```python
from build123d import *

# Parameters (mm, degrees)
F1_DEPTH  = 7.89
F3_DEPTH  = 9
F4_R      = 1.55
F5_DEPTH  = 25
F6_DEPTH  = 33
F7_R      = 2.53
F7_R_2    = 1.55
F8_DEPTH  = 1.12
F10_DEPTH = 1.98
F11_W     = 5.31
F11_H     = 0.8
F12_DEPTH = 1
F13_W     = 4.8969178084
F13_H     = 5.51
F14_DEPTH = 5.97
F15_R     = 2.46
F16_DEPTH = 2.5


with BuildPart() as f1:
    # F0 (on Front) → F1 (new body)
    with BuildSketch(Plane.XZ):
        Polygon((0, 10.28), (0, 1.53), (1.3, 1.53), (1.3, 2.33), (6.61, 2.33), (6.61, 1.53), (7.91, 1.53), (7.91, 10.28), align=None)
    extrude(amount=F1_DEPTH)

    # F2 (on face) → F3 (join)
    with BuildSketch(Plane.XZ.offset(7.89)):
        Polygon((1.3, 1.53), (0, 1.53), (0, 0), (7.91, 0), (7.91, 1.53), (6.61, 1.53), align=None)
    extrude(amount=-F3_DEPTH)

    # F4 (on face) → F5 (join)
    with BuildSketch(Plane(origin=(0, 0, 0), x_dir=(-1, 0, 0), z_dir=(0, 1, 0))):
        with Locations((-3.955, 6.065)):
            Circle(F4_R)
    extrude(amount=F5_DEPTH)

    # F6 (cut): a face of the model
    f6_faces = [f1.faces().sort_by_distance(p)[0] for p in [
        (3.955, 25, 6.065),
    ]]
    extrude(f6_faces, amount=-F6_DEPTH, mode=Mode.SUBTRACT)

    # F7 (on face) → F8 (join)
    with BuildSketch(Plane(origin=(0, 0, 0), x_dir=(-1, 0, 0), z_dir=(0, 1, 0))):
        with Locations((-3.955, 6.065)):
            Circle(F7_R)
        with Locations((-3.955, 6.065)):
            Circle(F7_R_2, mode=Mode.SUBTRACT)
    extrude(amount=F8_DEPTH)

    # F9 (on face) → F10 (join)
    with BuildSketch(Plane.XY.offset(10.28)):
        with BuildLine():
            ThreePointArc((3.955, 0), (2.487753429, -3.542246571), (6.03, -2.075))
            ThreePointArc((6.03, -2.075), (5.422246571, -0.607753429), (3.955, 0))
        make_face()
    extrude(amount=F10_DEPTH)

    # F11 (on face) → F12 (join)
    with BuildSketch(Plane.XZ.offset(7.89)):
        with Locations((3.955, 1.93)):
            Rectangle(F11_W, F11_H)
    extrude(amount=-F12_DEPTH)

    # F13 (on face) → F14 (cut)
    with BuildSketch(Plane.XZ.offset(7.89)):
        with Locations((3.955, 5.935)):
            Rectangle(F13_W, F13_H)
    extrude(amount=-F14_DEPTH, mode=Mode.SUBTRACT)

    # F15 (on face) → F16 (cut)
    with BuildSketch(Plane(origin=(0, 0, 0), x_dir=(1, 0, 0), z_dir=(0, 0, -1))):
        with Locations((3.955, 3.39)):
            Circle(F15_R)
    extrude(amount=-F16_DEPTH, mode=Mode.SUBTRACT)


solid = f1.part
```
The model under review builds one solid part; all positions refer to its coordinate system, in mm. A direction names the side the tool comes from. Round coordinates to 2 decimals unless told otherwise and drop trailing zeros. Write each loop counter-clockwise with the first axis right and the second up, starting at its lowest first coordinate (ties: lowest second). Pieces come first, ordered by that corner, then holes.
(1) We need section C-C on z = 1. Give the boundary of the cut face in (x, y) (3 decimals).
(2) Insertion check: pin 1 (1 mm diameter, centred on x = 7, y = 0, fed in from +Z); pin 2 (3.5 mm diameter, centred on x = 3.955, z = 6.065, fed in from -Y); pin 3 (1.5 mm diameter, centred on x = 4, z = 10.5, fed in from +Y). Each pin has a flat end and moves straight along its axis. Give the tip position at first contact, or say it passes through.
(3) We need section B-B on y = 0.5. Give the boundary of the cut face in (x, z) (3 decimals), and give its area (3 significant figures).
(4) Wall thickness on L1, parallel to Z at x = 2.25, y = -6.5; L2, parallel to X at y = -2, z = 1.75; L3, parallel to X at y = -3.39, z = 0.9 (3 decimals): over which ranges is each line inside the solid? List them lowest first.
(5) We need section D-D on y = -6.75. Give the boundary of the cut face in (x, z).
(6) We need section A-A on x = 4.25. Give the number of separate pieces and of enclosed holes in the cut face, and give its area (3 significant figures).
(7) Machinability: for faces 1 (the flat face through (2.8, -1.92, 4.7)), 2 (the flat face through (1, -3, 0)), 3 (the flat face through (4, -2, 12.26)), 4 (the cylindrical face through (6.3, -4.13, 0.75)), 5 (the flat face through (2, 0, 8)), which of the approach directions +Z, -Z, +X, -X, +Y, -Y give a long, thin tool a straight path to every point of the face, cutting with its end or side? Answer none if there is none.
(8) Mouldability with a two-part tool opening along X and no side actions: class faces 6 (the flat face through (4, -7.89, 3)), 7 (the cylindrical face through (1.618, 0.552, 5.096)), 8 (the flat face through (4, -5, 8.69)) as +X half, -X half, draft (parallel to the pull), parting line (faces both ways), or undercut.
Findings below:
1. outline: (0, -7.89) - (7.91, -7.89) - (7.91, 1.11) - (0, 1.11) - close; hole circle Ø4.92 at (3.955, -3.39)
2. pin 1: stops at z = 10.28
2. pin 2: stops at y = -1.92
2. pin 3: stops at y = 0
3. outline: (0, 0) - (7.91, 0) - (7.91, 1.53) - (0, 1.53) - close; circle Ø5.06 at (3.955, 6.065); hole circle Ø3.1 at (3.955, 6.065)
3. area: 24.7 mm2
4. L1: z = 0 to 1.53, 2.33 to 3.18, 8.69 to 10.28
4. L2: x = 0 to 1.3, 6.61 to 7.91
4. L3: x = 0 to 1.495, 6.415 to 7.91
5. outline: (0, 0) - (7.91, 0) - (7.91, 10.28) - (0, 10.28) - close; hole (1.3, 1.53) - (6.61, 1.53) - (6.61, 2.33) - (1.3, 2.33) - close; hole (1.51, 3.18) - (6.4, 3.18) - (6.4, 8.69) - (1.51, 8.69) - close
6. separate pieces: 3
6. enclosed holes: 0
6. area: 40.6 mm2
7. face 1: -Y
7. face 2: -Z, +X, -X, +Y, -Y
7. face 3: +Z, +X, -X, +Y, -Y
7. face 4: -Z
7. face 5: +Y
8. face 6: draft
8. face 7: parting line
8. face 8: undercut
